from build123d import *

# Parameters (mm, degrees)
F0_W     = 57.15
F0_H     = 31.75
F1_DEPTH = 38.1
F3_DEPTH = 12.7
F5_DEPTH = 38.1
F7_DEPTH = 12.7


with BuildPart() as f1:
    # F0 (on Front) → F1 (new body)
    with BuildSketch(Plane.XZ):
        with Locations((28.575, 15.875)):
            Rectangle(F0_W, F0_H)
    extrude(amount=F1_DEPTH)

    # F2 (on face) → F3 (cut)
    with BuildSketch(Plane.XZ.offset(38.1)):
        Polygon((31.75, 0), (57.15, 0), (44.966862, 31.75), (18.606976, 31.75), align=None)
    extrude(amount=-F3_DEPTH, mode=Mode.SUBTRACT)

    # F4 (on face) → F5 (cut)
    with BuildSketch(Plane.XZ.offset(38.1)):
        Polygon((57.15, 0), (57.15, 31.75), (44.966862, 31.75), align=None)
    extrude(amount=-F5_DEPTH, mode=Mode.SUBTRACT)

    # F6 (on face) → F7 (cut)
    with BuildSketch(Plane(origin=(0, 0, 0), x_dir=(-1, 0, 0), z_dir=(0, 1, 0))):
        Polygon((-25.739651, 0), (-16.746279, 31.75), (-44.966862, 31.75), (-57.15, 0), align=None)
    extrude(amount=-F7_DEPTH, mode=Mode.SUBTRACT)


solid = f1.part
CAD build for the part. Positions are in the model's coordinates, mm. A direction names the side the tool comes from. Round coordinates to 2 decimals unless told otherwise and drop trailing zeros. Order: outer loops, then holes, each group sorted by start corner. A loop starts at its lowest first (then second) coordinate and runs counter-clockwise, first axis right, second up. Notation, with made-up numbers: (-3.75, -29.5) - (53.25, -29.5) arc R20 ccw to (53.25, -1.5) - close; hole circle Ø8 at (75, -21.5). An arc over 180 degrees is marked (long way). Return JSON: item names as keys, results as strings.
(1) Tool access for faces 1 (the face through (0, -19, 16)), 2 (the face through (37, -12.7, 16)), 3 (the face through (38, -25.4, 16)): list every direction of +Z, -Z, +X, -X, +Y, -Y with a clear straight run to the whole face (end or side of a thin tool).
Answer key:
{"face 1": "+Z, -Z, -X, +Y, -Y", "face 2": "+Z, +X, +Y", "face 3": "+Z, +X, -Y"}
(2) Cut at B-B (z = 22). Give the cut face in (x, y).
Answer key:
{"outline": "(0, -38.1) - (22.64, -38.1) - (22.64, -25.4) - (48.71, -25.4) - (48.71, -12.7) - (19.51, -12.7) - (19.51, 0) - (0, 0) - close"}
(3) Wall check: probe 1 along Y at (x, z) = (22, 29); probe 2 along X at (y, z) = (-33, 15); probe 3 along X at (y, z) = (-6, 29). Give the ranges that are in metal, low to high. Write a range as from..to.
Answer key:
{"probe 1": "y = -25.4..-12.7", "probe 2": "x = 0..25.54", "probe 3": "x = 0..17.53"}
(4) Pin check, flat tips, straight feed: pin 1 Ø6 at (y, z) = (-25, 27) entering from +X; pin 2 Ø1 at (x, z) = (26, 23) entering from -Y; pin 3 Ø8 at (x, z) = (48.5, 7.5) entering from +Y. Stop position of each tip, or through.
Answer key:
{"pin 1": "stops at x = 47.94", "pin 2": "stops at y = -25.4", "pin 3": "stops at y = -12.7"}
(5) Cut at D-D (z = 4). Give the cut face in (x, y).
Answer key:
{"outline": "(0, -38.1) - (30.09, -38.1) - (30.09, -25.4) - (55.62, -25.4) - (55.62, -12.7) - (24.61, -12.7) - (24.61, 0) - (0, 0) - close"}
(6) Cut at C-C (y = -11.5). Give the cut face in (x, z).
Answer key:
{"outline": "(0, 0) - (25.74, 0) - (16.75, 31.75) - (0, 31.75) - close"}
(7) Cut at A-A (x = 37). Give the cut face in (y, z).
Answer key:
{"outline": "(-25.4, 0) - (-12.7, 0) - (-12.7, 31.75) - (-25.4, 31.75) - close"}
